Drawing for the job (mm, zero at the part's lowest x, y, z). Coordinates: 2 decimals unless noted, no trailing zeros. Answer as CSV lines item,"result".
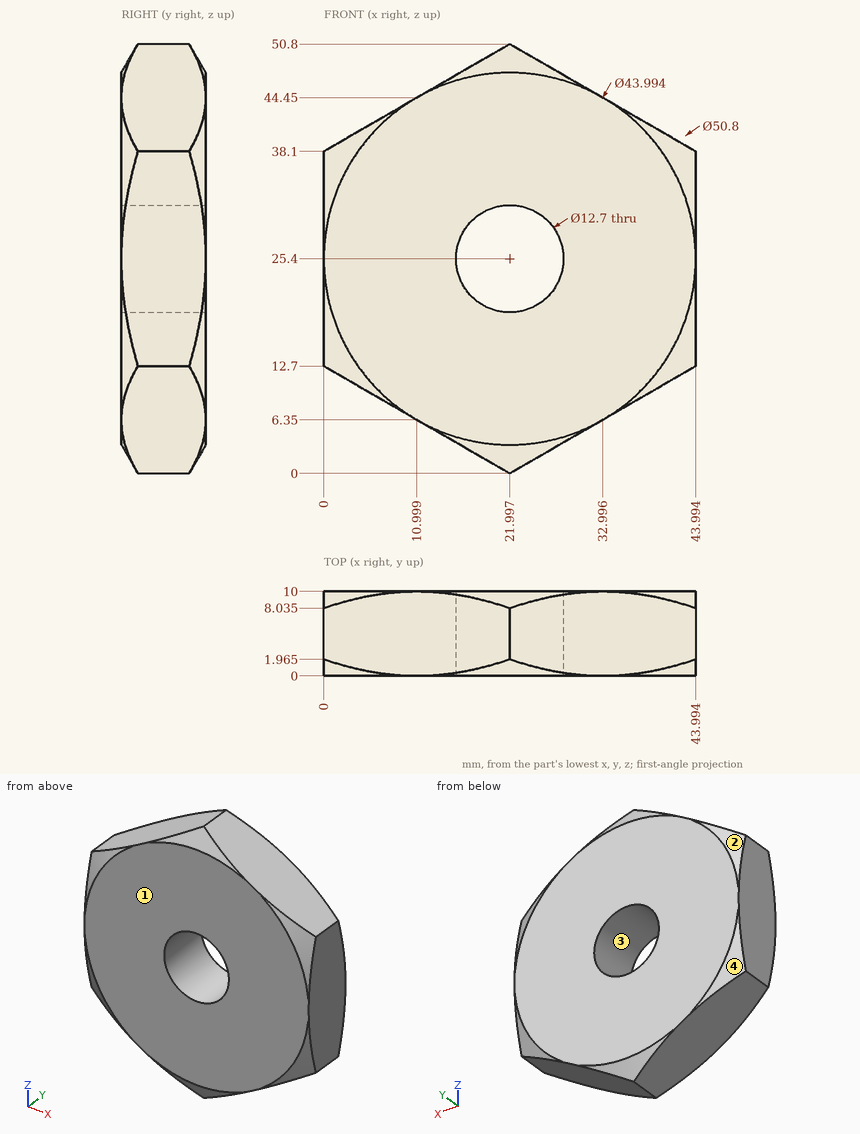
Item 1: Wall check: line 1 (X direction, y = 3.5, z = 24) (1 decimal); line 2 (Z direction, x = 21, y = 8.5) (1 decimal); line 3 (Z direction, x = 23, y = 9.5) (1 decimal). Give the ranges that are in metal, low to high. Write a range as from..to.
Answer below:
line 1,"x = 0..15.8, 28.2..44"
line 2,"z = 0.8..19.1, 31.7..50"
line 3,"z = 2.6..19.1, 31.7..48.2"
Item 2: Two-plate mould, pull along Z, no slides. Class the marked faces 1, 2, 3 and 4: pulls with the +Z half, pulls with the -Z half, needs draft (parallel to the pull), parting line crosses it, or undercut.
Answer below:
face 1,"needs draft"
face 2,"pulls with the +Z half"
face 3,"undercut"
face 4,"pulls with the -Z half"
Item 3: Flat gauge pins, fed straight in: pin 1 (5 mm diameter, centred on x = 18.5, y = 4, fed in from -Z) (1 decimal); pin 2 (7.5 mm diameter, centred on x = 22, z = 25.4, fed in from -Y); pin 3 (1 mm diameter, centred on x = 25.5, y = 2, fed in from -Z) (1 decimal); pin 4 (5 mm diameter, centred on x = 5.5, y = 5.5, fed in from -Z). Where does each tip first touch, or does it go through?
Answer below:
pin 1,"stops at z = 0.6"
pin 2,"passes through"
pin 3,"stops at z = 1.7"
pin 4,"stops at z = 8.08"
